The model under review builds one solid part; all positions refer to its coordinate system, in mm. Face numbers are marked on the shaded views. A direction names the side the tool comes from. Round coordinates to 2 decimals unless told otherwise and drop trailing zeros. Write each loop counter-clockwise with the first axis right and the second up, starting at its lowest first coordinate (ties: lowest second). Pieces come first, ordered by that corner, then holes. Notation, with made-up numbers: (80, 11) - (85, 11) arc R15 cw to (85, 22) - close; hole circle Ø4 at (-6.5, 69). An arc over 180 degrees is marked (long way). Use one line per item in the form item = value.
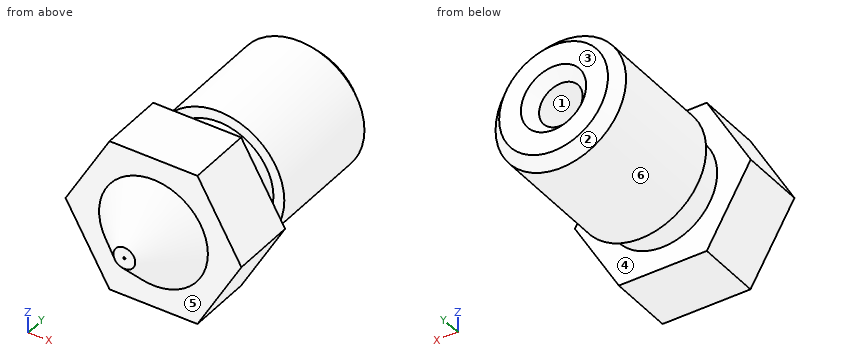
from build123d import *

# Parameters (mm, degrees)
BOSS_EXTRUDE1_DEPTH = 3
CHAMFER1_SIZE       = 0.5


with BuildPart() as part:
    # Sketch1 → Boss-Extrude1 (new body)
    with BuildSketch(Plane.XZ):
        Polygon((-2.020725942, 3.5), (-4.041451884, 0), (-2.020725942, -3.5), (2.020725942, -3.5), (4.041451884, 0), (2.020725942, 3.5), align=None)
    extrude(amount=-BOSS_EXTRUDE1_DEPTH)

    # Sketch2 → Revolve1 (revolve)
    with BuildSketch(Plane(origin=(0, 0, 0), x_dir=(-1, 0, 0), z_dir=(0, 0, -1))):
        Polygon((-2.5, 3), (0, 3), (0, 10.5), (-3, 10.5), (-3, 4.5), (-2.5, 4.5), align=None)
    revolve(axis=Axis((0, 3, 0), (0, 1, 0)))

    # Sketch3 → Revolve2 (revolve)
    with BuildSketch(Plane.XY):
        Polygon((2.5, 0), (0, 0), (0, -2), (0.5, -2), align=None)
    revolve(axis=Axis((0, 0, 0), (0, -1, 0)))

    # Sketch4 → Cut-Revolve1 (revolve, cut)
    with BuildSketch(Plane(origin=(0, 0, 0), x_dir=(-1, 0, 0), z_dir=(0, 0, -1))):
        Polygon((-0.05, -2), (0, -2), (0, 10.5), (-1, 10.5), (-1, 0), (-0.75, -0.227272727), (-0.75, -0.7), (-0.05, -1.2), align=None)
    revolve(axis=Axis((0, -2, 0), (0, 1, 0)), mode=Mode.SUBTRACT)

    # Chamfer1
    chamfer1_edges = [part.edges().sort_by_distance(p)[0] for p in [
        (-3, 10.5, 0),
        (-1, 10.5, 0),
    ]]
    chamfer(chamfer1_edges, length=CHAMFER1_SIZE)


solid = part.part
(1) Add section A-A on y = 0.5. Write out the cut boundary in (x, z).
Geometry results:
outline = (-4.04, 0) - (-2.02, -3.5) - (2.02, -3.5) - (4.04, 0) - (2.02, 3.5) - (-2.02, 3.5) - close; hole circle Ø2 at (0, 0)
(2) Add section D-D on y = 3.5. Write out the cut boundary in (x, z).
Geometry results:
outline = circle Ø5 at (0, 0); hole circle Ø2 at (0, 0)
(3) The part is to be moulded in two halves that separate along Z. For the marked faces 1, 2 and 3, say which applies: +Z half, -Z half, draft (parallel to the pull), parting line (faces both ways), or undercut.
Geometry results:
face_1 = undercut
face_2 = parting line
face_3 = draft
(4) Machinability: for the marked faces 4, 5 and 6, which of the approach directions +Z, -Z, +X, -X, +Y, -Y give a long, thin tool a straight path to every point of the face, cutting with its end or side? Answer none if there is none.
Geometry results:
face_4 = none
face_5 = -Y
face_6 = +Y
(5) To check wall thickness, follow L1, parallel to X at y = 4.75, z = 0; L2, parallel to Z at x = 0, y = 2.25; L3, parallel to X at y = 3.75, z = 0. State the ranges of each line that lie inside material, in increasing order.
Geometry results:
L1 = -3 to -1, 1 to 3
L2 = -3.5 to -1, 1 to 3.5
L3 = -2.5 to -1, 1 to 2.5
(6) Add section C-C on x = -3.25. Write out the cut boundary in (y, z), then the cut area to 4 significant figures.
Geometry results:
outline = (0, -1.37) - (3, -1.37) - (3, 1.37) - (0, 1.37) - close
area = 8.225 mm2
(7) Add section B-B on y = 7.5. Write out the cut boundary in (x, z).
Geometry results:
outline = circle Ø6 at (0, 0); hole circle Ø2 at (0, 0)
(8) Insertion check: P1, Ø1.8, axis at x = 0, z = 0, coming from the +Y side; P2, Ø1, axis at x = 1.5, z = 2.5, coming from the -Y side. Each pin has a flat end and moves straight along its axis. Give the tip position at first contact, or say it passes through.
Geometry results:
P1 = -0.09
P2 = -0.08
